Geometry: see drawing. Coordinates: mm, zero at the bounding-box minimum. Round coordinates to 2 decimals unless told otherwise and drop trailing zeros. Write each loop counter-clockwise with the first axis right and the second up, starting at its lowest first coordinate (ties: lowest second). Pieces come first, ordered by that corner, then holes.
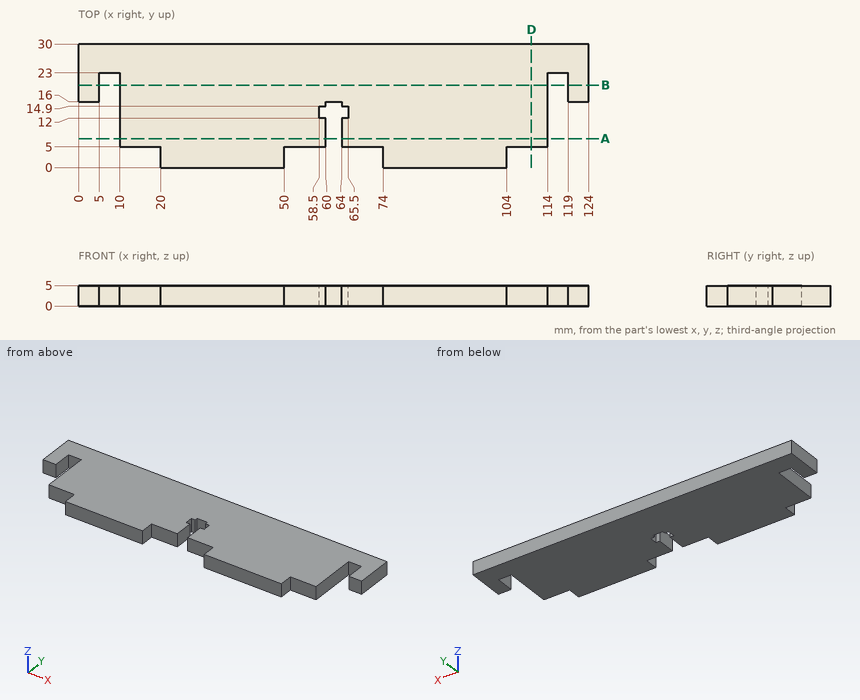
Q1. Section query A-A, the plane y = 7. Output: boundary loops of the cut face in (x, z).
Q2. Section query D-D, the plane x = 110. Output: boundary loops of the cut face in (y, z).
Q3. Section query B-B, the plane y = 20. Output: boundary loops of the cut face in (x, z), and give its area (3 significant figures).
Q4. Pin query (flat end, axial travel): P1, Ø0.9, axis at y = 13, z = 1.5, coming from the +X side; P2, Ø0.5, axis at y = 15.5, z = 2, coming from the -X side. Return the tip coordinate at first contact, or that it passes through.
Q5. Line query: line 1 (X direction, y = 22.5, z = 3.75); line 2 (X direction, y = 6.25, z = 1.8); line 3 (X direction, y = 13.75, z = 1.75). Output: solid intervals per line, ascending.
Filled in:
1. outline: (10, 0) - (60, 0) - (60, 5) - (10, 5) - close; (64, 0) - (114, 0) - (114, 5) - (64, 5) - close
2. outline: (5, 0) - (30, 0) - (30, 5) - (5, 5) - close
3. outline: (0, 0) - (5, 0) - (5, 5) - (0, 5) - close; (10, 0) - (114, 0) - (114, 5) - (10, 5) - close; (119, 0) - (124, 0) - (124, 5) - (119, 5) - close
3. area: 570 mm2
4. P1: stops at x = 114
4. P2: stops at x = 10
5. line 1: x = 0 to 5, 10 to 114, 119 to 124
5. line 2: x = 10 to 60, 64 to 114
5. line 3: x = 10 to 58.5, 65.5 to 114
